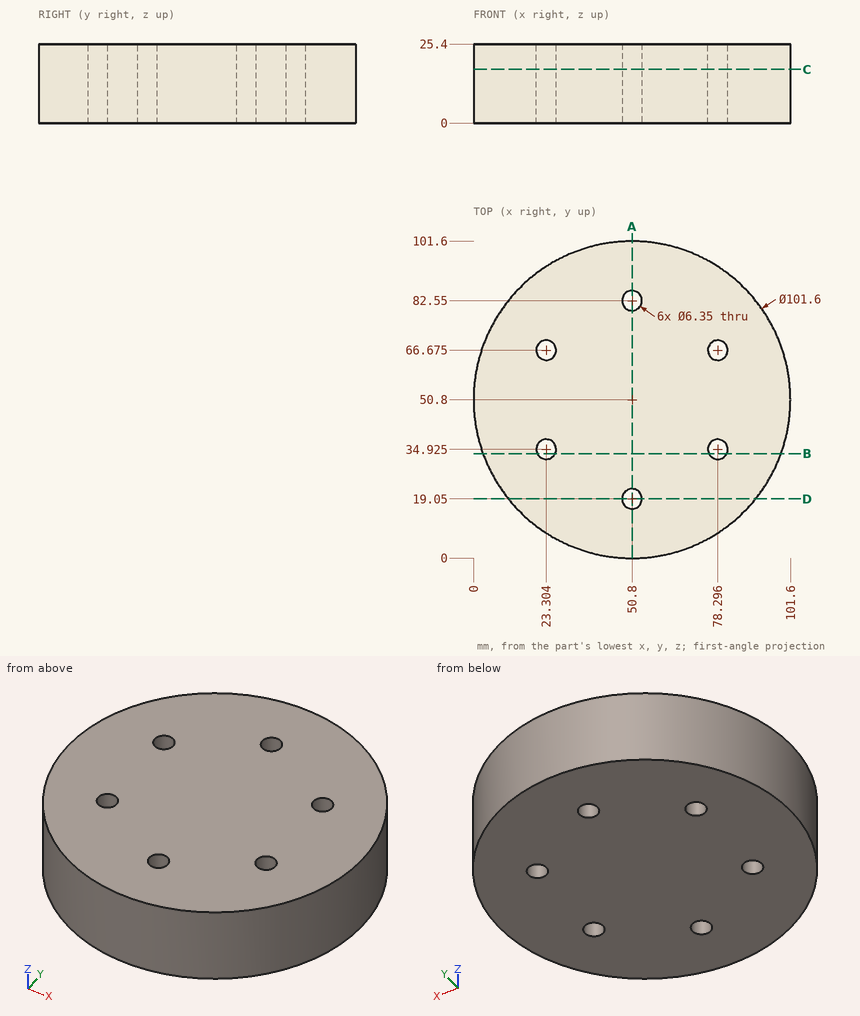
Answer from the drawing. Dimensions are ordinates in mm from the lowest x, y and z of the part. Round coordinates to 2 decimals unless told otherwise and drop trailing zeros. Write each loop counter-clockwise with the first axis right and the second up, starting at its lowest first coordinate (ties: lowest second). Pieces come first, ordered by that corner, then holes. Notation, with made-up numbers: (-28.5, 16.5) -> (-3.5, 16.5) arc R20 ccw to (-3.5, 21.5) -> close; hole circle Ø11 at (65, 2). An arc over 180 degrees is marked (long way). Answer in a Markdown table with one row per item. Add a question column.
1) Consider line 1 (Y direction, x = 50.8, z = 13.75) (1 decimal); line 2 (Y direction, x = 79.5, z = 11) (1 decimal); line 3 (X direction, y = 82.55, z = 16) (1 decimal). Determine where each line is inside the solid, lowest interval first.
2) Find section A-A, the plane x = 50.8. Determine the outline of the cut face in (y, z) (1 decimal), and give its area (3 significant figures).
3) Given P1, Ø1, axis at y = 46.5, z = 6.5, coming from the -X side; P2, Ø4, axis at x = 23.3, y = 34.92, coming from the +Z side; P3, Ø5, axis at y = 67.5, z = 8, coming from the +X side (1 decimal); P4, Ø8.5, axis at x = 78.3, y = 34.92, coming from the -Z side, each flat-ended and moving along its own axis, determine where each tip first touches the part or whether it passes through.
4) Find section C-C, the plane z = 17.25. State how many separate pieces and enclosed holes the cut face has, and give its area (3 significant figures).
5) Find section B-B, the plane y = 33.5. Determine the outline of the cut face in (x, z).
6) Find section D-D, the plane y = 19.05. Determine the outline of the cut face in (x, z) (1 decimal), and give its area (3 significant figures).
Findings below:
| question | item | result |
|---|---|---|
| 1 | line 1 | 0 to 15.9, 22.2 to 79.4, 85.7 to 101.6 |
| 1 | line 2 | 8.9 to 32, 37.9 to 63.7, 69.6 to 92.7 |
| 1 | line 3 | 11.1 to 47.6, 54 to 90.5 |
| 2 | outline | (0, 0) -> (15.9, 0) -> (15.9, 25.4) -> (0, 25.4) -> close; (22.2, 0) -> (79.4, 0) -> (79.4, 25.4) -> (22.2, 25.4) -> close; (85.7, 0) -> (101.6, 0) -> (101.6, 25.4) -> (85.7, 25.4) -> close |
| 2 | area | 2,260 mm² |
| 3 | P1 | x = 0.14 |
| 3 | P2 | through |
| 3 | P3 | x = 99.6 |
| 3 | P4 | z = 0 |
| 4 | separate pieces | 1 |
| 4 | enclosed holes | 6 |
| 4 | area | 7,920 mm² |
| 5 | outline | (3.04, 0) -> (20.47, 0) -> (20.47, 25.4) -> (3.04, 25.4) -> close; (26.14, 0) -> (75.46, 0) -> (75.46, 25.4) -> (26.14, 25.4) -> close; (81.13, 0) -> (98.56, 0) -> (98.56, 25.4) -> (81.13, 25.4) -> close |
| 6 | outline | (11.1, 0) -> (47.6, 0) -> (47.6, 25.4) -> (11.1, 25.4) -> close; (54, 0) -> (90.5, 0) -> (90.5, 25.4) -> (54, 25.4) -> close |
| 6 | area | 1,850 mm² |
